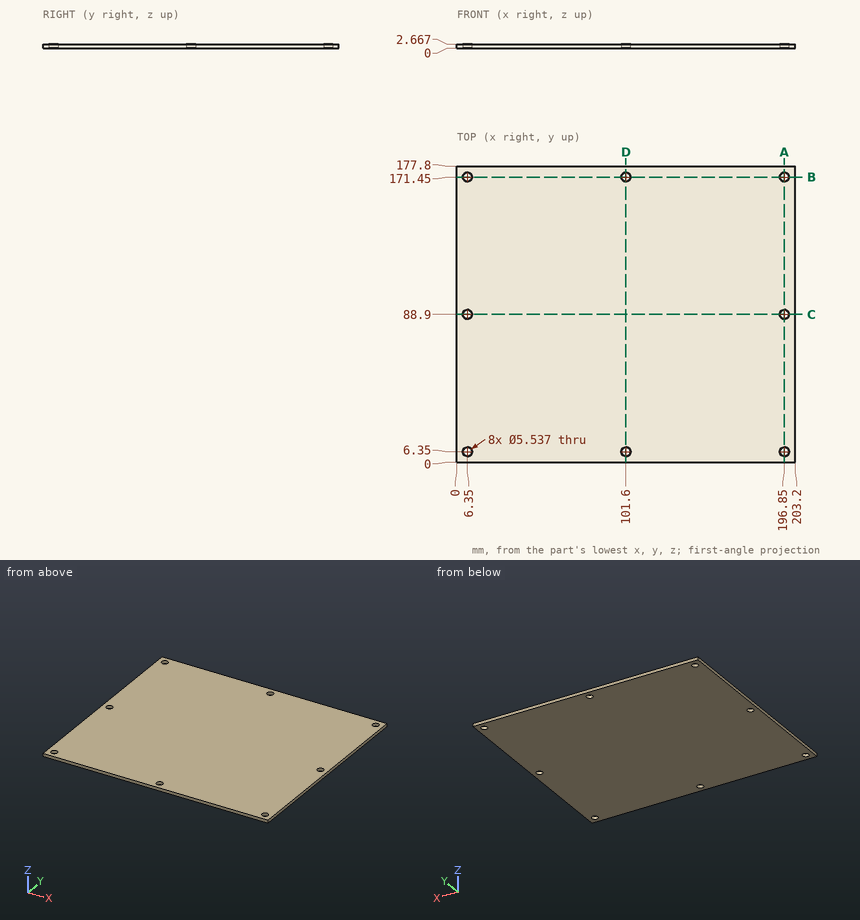
Geometry: see drawing. Coordinates: mm, zero at the bounding-box minimum. Give positions to 0.01 mm unless a question says otherwise; leave off trailing zeros. Loops run counter-clockwise (first coordinate to the right, second up) from the corner with the lowest first, then second, coordinate; pieces in that order, holes last. Notation, with made-up numbers: (34, 69.5) - (56, 69.5) arc R26 ccw to (56, 94.5) - close; hole circle Ø10 at (0, 28). An arc over 180 degrees is marked (long way). Answer as CSV lines item,"result". Start each with the question number.
1. Section B-B, the plane y = 171.45. Return loops of the section in (x, z).
2. Section A-A, the plane x = 196.85. Return loops of the section in (y, z), plus the area to 3 significant figures.
3. Pin query (flat end, axial travel): P1, Ø1, axis at y = 101, z = 1.5, coming from the -X side. Return the tip coordinate at first contact, or that it passes through.
4. Section C-C, the plane y = 88.9. Return loops of the section in (x, z).
5. Section D-D, the plane x = 101.6. Return loops of the section in (y, z), plus the area to 3 significant figures.
6. Ray query, L1, parallel to X at y = 6.35, z = 1.7; L2, parallel to X at y = 88.9, z = 1.8; L3, parallel to Y at x = 196.85, z = 1.95. Return the intervals inside material, ascending.
Answers:
1,outline,"(0, 0) - (3.58, 0) - (3.58, 2.67) - (0, 2.67) - close; (9.12, 0) - (98.83, 0) - (98.83, 2.67) - (9.12, 2.67) - close; (104.37, 0) - (194.08, 0) - (194.08, 2.67) - (104.37, 2.67) - close; (199.62, 0) - (203.2, 0) - (203.2, 2.67) - (199.62, 2.67) - close"
2,outline,"(0, 0) - (3.58, 0) - (3.58, 2.67) - (0, 2.67) - close; (9.12, 0) - (86.13, 0) - (86.13, 2.67) - (9.12, 2.67) - close; (91.67, 0) - (168.68, 0) - (168.68, 2.67) - (91.67, 2.67) - close; (174.22, 0) - (177.8, 0) - (177.8, 2.67) - (174.22, 2.67) - close"
2,area,"430 mm2"
3,P1,"stops at x = 0"
4,outline,"(0, 0) - (3.58, 0) - (3.58, 2.67) - (0, 2.67) - close; (9.12, 0) - (194.08, 0) - (194.08, 2.67) - (9.12, 2.67) - close; (199.62, 0) - (203.2, 0) - (203.2, 2.67) - (199.62, 2.67) - close"
5,outline,"(0, 0) - (3.58, 0) - (3.58, 2.67) - (0, 2.67) - close; (9.12, 0) - (168.68, 0) - (168.68, 2.67) - (9.12, 2.67) - close; (174.22, 0) - (177.8, 0) - (177.8, 2.67) - (174.22, 2.67) - close"
5,area,"445 mm2"
6,L1,"x = 0 to 3.58, 9.12 to 98.83, 104.37 to 194.08, 199.62 to 203.2"
6,L2,"x = 0 to 3.58, 9.12 to 194.08, 199.62 to 203.2"
6,L3,"y = 0 to 3.58, 9.12 to 86.13, 91.67 to 168.68, 174.22 to 177.8"
